Input: dimensioned drawing with shaded views. Units: mm. Origin: part minimum x, y, z. A direction names the side the tool comes from. Round coordinates to 2 decimals unless told otherwise and drop trailing zeros. Write each loop counter-clockwise with the first axis right and the second up, starting at its lowest first coordinate (ties: lowest second). Pieces come first, ordered by that corner, then holes. Notation, with made-up numbers: M -29,22.5 L -23,22.5 A16 cw -23,44.5 Z; hole C 62.25,72 d11. An arc over 180 degrees is marked long. Use one line per item in the form item = value. Start each with the question number.
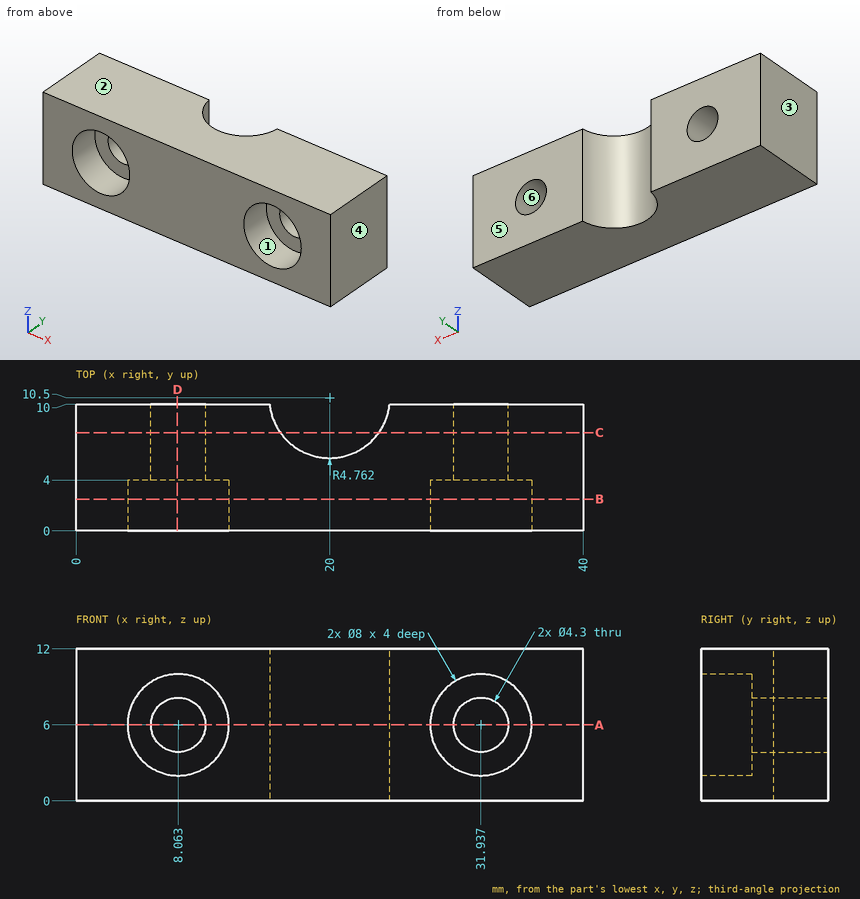
1. Section query D-D (x = 8). Return loops of the section in (y, z).
2. Ray query, probe 1 along X at (y, z) = (3.25, 2.5) (1 decimal); probe 2 along X at (y, z) = (9.25, 4.75) (1 decimal); probe 3 along Y at (x, z) = (30, 8.75). Return the intervals inside material, ascending.
3. Pull-direction query (X, two-part tool) for the marked faces 3, 4, 5 and 6; classes: released by +X, released by -X, zero draft, split by the parting line, or undercut.
4. Section query A-A (z = 6). Return loops of the section in (x, y) (1 decimal).
5. Section query C-C (y = 7.75). Return loops of the section in (x, z).
6. Section query B-B (y = 2.5). Return loops of the section in (x, z).
7. Contact query for flat-ended pins moving along their axis: pin 1 (2.5 mm diameter, centred on x = 7, z = 6.5, fed in from -Y); pin 2 (3.5 mm diameter, centred on x = 8.06, z = 6, fed in from -Y). Output: stop coordinate, or through.
8. Set-up query: the marked faces 1 and 2. Return all of +Z, -Z, +X, -X, +Y, -Y with unobstructed straight access to the full face (end or side cutting, diameter ignored); none if empty.
Checks:
q1.outline = M 0,0 L 10,0 L 10,3.85 L 4,3.85 L 4,2 L 0,2 Z; M 0,10 L 4,10 L 4,8.15 L 10,8.15 L 10,12 L 0,12 Z
q2.probe_1 = 0 to 6.1, 10 to 30, 33.9 to 40
q2.probe_2 = 0 to 6.3, 9.8 to 15.4, 24.6 to 30.2, 33.7 to 40
q2.probe_3 = 4 to 10
q3.face_3 = released by -X
q3.face_4 = released by +X
q3.face_5 = zero draft
q3.face_6 = undercut
q4.outline = M 0,0 L 4.1,0 L 4.1,4 L 5.9,4 L 5.9,10 L 0,10 Z; M 10.2,4 L 12.1,4 L 12.1,0 L 27.9,0 L 27.9,4 L 29.8,4 L 29.8,10 L 24.7,10 A4.8 cw 15.3,10 L 10.2,10 Z; M 34.1,4 L 35.9,4 L 35.9,0 L 40,0 L 40,10 L 34.1,10 Z
q5.outline = M 0,0 L 16.11,0 L 16.11,12 L 0,12 Z; M 23.89,0 L 40,0 L 40,12 L 23.89,12 Z; hole C 8.06,6 d4.3; hole C 31.94,6 d4.3
q6.outline = M 0,0 L 40,0 L 40,12 L 0,12 Z; hole C 8.06,6 d8; hole C 31.94,6 d8
q7.pin_1 = 4
q7.pin_2 = through
q8.face_1 = -Y
q8.face_2 = +Z, +X, -X, +Y, -Y
